Read the model definition and answer for the solid it produces. Units are mm, in the model's axes. Face numbers are marked on the shaded views. Round coordinates to 2 decimals unless told otherwise and drop trailing zeros. Order: outer loops, then holes, each group sorted by start corner. A loop starts at its lowest first (then second) coordinate and runs counter-clockwise, first axis right, second up. Notation, with made-up numbers: M 1,20.25 L 54,20.25 A23 ccw 54,50.25 Z; hole C 18,82 d5. An arc over 180 degrees is marked long. Use one line per item in the form item = value. Start each with the question number.
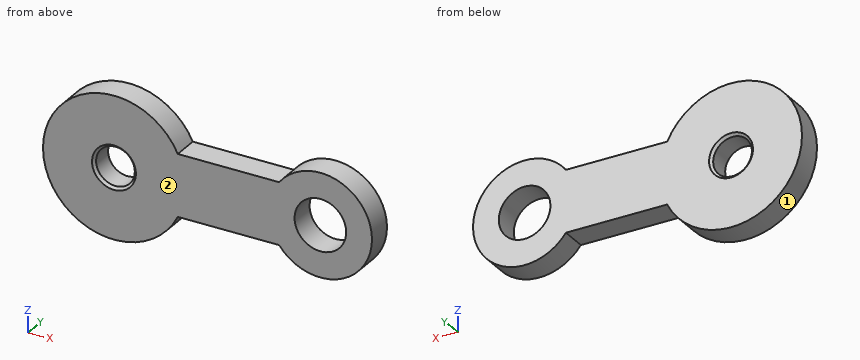
from build123d import *

# Parameters (mm, degrees)
SKETCH1_R           = 9.525
SKETCH1_R_2         = 12.7
BOSS_EXTRUDE1_DEPTH = 12.7
CHAMFER1_SIZE       = 1.27


with BuildPart() as part:
    # Sketch1 → Boss-Extrude1 (new body)
    with BuildSketch(Plane(origin=(0, 0, 0), x_dir=(1, 0, 0), z_dir=(0, 1, 0))):
        with BuildLine():
            Line((31.4244813, 15.24), (81.28, 15.24))
            ThreePointArc((81.28, 15.24), (127, 0), (81.28, -15.24))
            Line((81.28, -15.24), (31.4244813, -15.24))
            ThreePointArc((31.4244813, -15.24), (-34.925, 0), (31.4244813, 15.24))
        make_face()
        with Locations(Location((0, 0, 0), (0, 0, 270))):
            Circle(SKETCH1_R, mode=Mode.SUBTRACT)
        with Locations(Location((101.6, 0, 0), (0, 0, 270))):
            Circle(SKETCH1_R_2, mode=Mode.SUBTRACT)
    extrude(amount=BOSS_EXTRUDE1_DEPTH)

    # Chamfer1
    chamfer1_edges = [part.edges().sort_by_distance(p)[0] for p in [
        (0, 0, -9.525),
        (0, 12.7, -9.525),
    ]]
    chamfer(chamfer1_edges, length=CHAMFER1_SIZE)


solid = part.part
Item 1: For a pull along X with two mould halves and no side action, classify the marked faces 1 and 2 as pulls with the +X half, pulls with the -X half, needs draft (parallel to the pull), parting line crosses it, or undercut.
Item 2: Given P1, Ø1, axis at x = -6.5, y = 8, coming from the -Z side; P2, Ø5, axis at x = -11, y = 4.5, coming from the -Z side; P3, Ø4, axis at x = 110, y = 8, coming from the +Z side; P4, Ø23, axis at x = 101.6, z = 0, coming from the -Y side, each flat-ended and moving along its own axis, determine where each tip first touches the part or whether it passes through.
Item 3: Section B-B (x = 101.6) is taken. Write down the section's boundary in (y, z), and give its area (3 significant figures).
Item 4: Section D-D (x = 0) is taken. Write down the section's boundary in (y, z) (3 decimals).
Item 5: Section C-C (y = 5.5) is taken. Write down the section's boundary in (x, z) (3 decimals), and give its area (3 significant figures).
Item 6: Section A-A (z = 0) is taken. Write down the section's boundary in (x, y) (3 decimals), and give its area (3 significant figures).
Item 7: Find the intervals of material crossed by L1, parallel to X at y = 3.5, z = 6; L2, parallel to X at y = 8.5, z = -4; L3, parallel to Z at x = -24, y = 6.75, in increasing order. Write a range as [from, to].
The answers:
q1.face_1 = undercut
q1.face_2 = needs draft
q2.P1 = -34.41
q2.P2 = -33.87
q2.P3 = 24.58
q2.P4 = through
q3.outline = M 0,-25.4 L 12.7,-25.4 L 12.7,-12.7 L 0,-12.7 Z; M 0,12.7 L 12.7,12.7 L 12.7,25.4 L 0,25.4 Z
q3.area = 323 mm²
q4.outline = M 0,-34.925 L 12.7,-34.925 L 12.7,-10.795 L 11.43,-9.525 L 1.27,-9.525 L 0,-10.795 Z; M 0,10.795 L 1.27,9.525 L 11.43,9.525 L 12.7,10.795 L 12.7,34.925 L 0,34.925 Z
q5.outline = M 31.424,-15.24 L 81.28,-15.24 A25.4 ccw long 81.28,15.24 L 31.424,15.24 A34.925 ccw long Z; hole C 0,0 d19.05; hole C 101.6,0 d25.4
q5.area = 6,410 mm²
q6.outline = M -34.925,0 L -10.795,0 L -9.525,1.27 L -9.525,11.43 L -10.795,12.7 L -34.925,12.7 Z; M 9.525,1.27 L 10.795,0 L 88.9,0 L 88.9,12.7 L 10.795,12.7 L 9.525,11.43 Z; M 114.3,0 L 127,0 L 127,12.7 L 114.3,12.7 Z
q6.area = 1,490 mm²
q7.L1 = [-34.41, -7.4], [7.4, 90.41], [112.79, 126.28]
q7.L2 = [-34.7, -8.64], [8.64, 89.55], [113.65, 126.68]
q7.L3 = [-25.37, 25.37]
